Geometry: final body of the model. Coordinates: model frame, mm. Face numbers are marked on the shaded views. Give positions to 0.01 mm unless a question says otherwise; leave off trailing zeros. Write each loop counter-clockwise with the first axis right and the second up, starting at its lowest first coordinate (ties: lowest second). Pieces come first, ordered by that corner, then holes. Notation, with made-up numbers: M 25.5,46 L 70.5,46 A18 cw 70.5,69 Z; hole C 61.5,55.25 d1. An arc over 180 degrees is marked long. Use a Markdown table: item, result. Add a question column.
(1) Cut plane C-C (z = 60). Output: boundary loops of the cut face in (x, y).
(2) Cut plane A-A (y = 184.15). Output: boundary loops of the cut face in (x, z).
(3) Material intervals for L1, parallel to Y at x = 0, z = 6.5; L2, parallel to Y at x = 0, z = 82.5; L3, parallel to Y at x = 9.5, z = 14, sorted ascending.
(4) Pin query (flat end, axial travel): pin 1 Ø5 at (x, z) = (-1, 48.5) entering from -Y; pin 2 Ø8 at (x, z) = (-46.5, 59.5) entering from -Y; pin 3 Ø8 at (x, z) = (-25.5, 21.5) entering from -Y. Return the tip coordinate at first contact, or that it passes through.
(5) Cut plane B-B (x = 0). Output: boundary loops of the cut face in (y, z), plus the area to 3 significant figures.
(6) Draft query along X for the marked faces 1, 2, 3 and 4. Return one class per face: released by +X, released by -X, zero draft, split by the parting line, or undercut.
(7) Cut plane D-D (y = -11). Output: boundary loops of the cut face in (x, z), plus the area to 3 significant figures.
```python
from build123d import *

# Parameters (mm, degrees)
SKETCH3_R           = 63.5
SKETCH3_R_2         = 25.4
BOSS_EXTRUDE1_DEPTH = 127
SKETCH4_R           = 25.4
SKETCH4_R_2         = 38.1
BOSS_EXTRUDE2_DEPTH = 25.4


with BuildPart() as part:
    # Sketch3 → Boss-Extrude1 (new body)
    with BuildSketch(Plane(origin=(0, 0, 0), x_dir=(0, 1, 0), z_dir=(0, 0, 1))):
        with Locations(Location((0, 0, 0), (0, 0, 270))):
            Circle(SKETCH3_R)
        with Locations(Location((0, 0, 0), (0, 0, 270))):
            Circle(SKETCH3_R_2, mode=Mode.SUBTRACT)
    extrude(amount=BOSS_EXTRUDE1_DEPTH)

    # Sketch4 → Boss-Extrude2 (add)
    with BuildSketch(Plane(origin=(0, 0, 0), x_dir=(0, 1, 0), z_dir=(0, 0, 1))):
        with BuildLine():
            Line((0, 63.5), (241.3, 63.5))
            Line((241.3, 63.5), (241.3, -63.5))
            Line((241.3, -63.5), (0, -63.5))
            ThreePointArc((0, -63.5), (-63.5, 0), (0, 63.5))
        make_face()
        with Locations(Location((0, 0, 0), (0, 0, 270))):
            Circle(SKETCH4_R, mode=Mode.SUBTRACT)
        with Locations(Location((184.15, 0, 0), (0, 0, 270))):
            Circle(SKETCH4_R_2, mode=Mode.SUBTRACT)
    extrude(amount=BOSS_EXTRUDE2_DEPTH)


solid = part.part
```
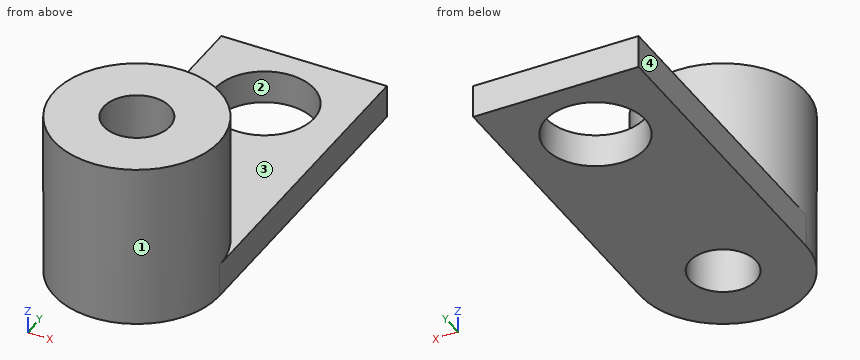
Answer list:
| question | item | result |
|---|---|---|
| 1 | outline | C 0,0 d127; hole C 0,0 d50.8 |
| 2 | outline | M -63.5,0 L -38.1,0 L -38.1,25.4 L -63.5,25.4 Z; M 38.1,0 L 63.5,0 L 63.5,25.4 L 38.1,25.4 Z |
| 3 | L1 | -63.5 to -25.4, 25.4 to 146.05, 222.25 to 241.3 |
| 3 | L2 | -63.5 to -25.4, 25.4 to 63.5 |
| 3 | L3 | -62.79 to -23.56, 23.56 to 147.25, 221.05 to 241.3 |
| 4 | pin 1 | y = -63.5 |
| 4 | pin 2 | y = -47.18 |
| 4 | pin 3 | y = -59.75 |
| 5 | outline | M -63.5,0 L -25.4,0 L -25.4,127 L -63.5,127 Z; M 25.4,0 L 146.05,0 L 146.05,25.4 L 63.5,25.4 L 63.5,127 L 25.4,127 Z; M 222.25,0 L 241.3,0 L 241.3,25.4 L 222.25,25.4 Z |
| 5 | area | 12,300 mm² |
| 6 | face 1 | split by the parting line |
| 6 | face 2 | undercut |
| 6 | face 3 | zero draft |
| 6 | face 4 | released by -X |
| 7 | outline | M -62.54,0 L -22.89,0 L -22.89,127 L -62.54,127 Z; M 22.89,0 L 62.54,0 L 62.54,127 L 22.89,127 Z |
| 7 | area | 10,100 mm² |
